Verification items for the finished model (mm, model axes). A direction names the side the tool comes from. Coordinates: 2 decimals unless noted, no trailing zeros. Write each loop counter-clockwise with the first axis right and the second up, starting at its lowest first coordinate (ties: lowest second). Pieces come first, ordered by that corner, then holes. Notation, with made-up numbers: M 50.5,21.5 L 97.5,21.5 A12 cw 97.5,30.5 Z; hole C 41.5,76 d4. An arc over 180 degrees is marked long. Answer in a Markdown table with one row per item.
from build123d import *

# Parameters (mm, degrees)
SKETCH1_W               = 0.625
SKETCH1_H               = 3.375
CUT_REVOLVE1_START      = -4.0000001
CUT_REVOLVE1_OUTLINE_R  = 0.625
CUT_REVOLVE1_DEPTH      = 4.6250001
SKETCH1_4_W             = 0.625
SKETCH1_4_H             = 3.375
SKETCH1_4_H_2           = 0.625
CUT_EXTRUDE1_DEPTH      = 20.584751879
CUT_EXTRUDE1_DEPTH_BACK = 20.584751879


# Read off the part's stored shape, not the designer's step: Cut-Revolve1
with BuildPart() as part:
    # Sketch1 → Revolve1 (revolve)
    with BuildSketch(Plane.XY):
        Polygon((18.75, 4), (16.875, 4), (16.875, 0.625), (16.875, 0), (18.75, 0), align=None)
        with Locations((16.5625, 2.3125)):
            Rectangle(SKETCH1_W, SKETCH1_H)
        Polygon((-18.75, 4), (-18.75, 0), (-16.875, 0), (-16.875, 0.625), (-0.625, 0.625), (0, 0.625), (16.25, 0.625), (16.25, 4), align=None)
    revolve(axis=Axis((0, 0, 0), (-1, 0, 0)))

    # Cut-Revolve1 outline → Cut-Revolve1 (cut)
    with BuildSketch(Plane(origin=(0, 0, 0), x_dir=(1, 0, 0), z_dir=(0, 1, 0)).offset(CUT_REVOLVE1_START)):
        Circle(CUT_REVOLVE1_OUTLINE_R)
    extrude(amount=CUT_REVOLVE1_DEPTH, mode=Mode.SUBTRACT)

    # Sketch1_4 → Cut-Revolve2 (revolve, cut)
    with BuildSketch(Plane.XY):
        with Locations((16.5625, 2.3125)):
            Rectangle(SKETCH1_4_W, SKETCH1_4_H)
        with Locations((16.5625, 0.3125)):
            Rectangle(SKETCH1_4_W, SKETCH1_4_H_2)
        with Locations((16.5625, -0.3125)):
            Rectangle(SKETCH1_4_W, SKETCH1_4_H_2)
    cut_revolve2 = revolve(axis=Axis((16.25, -0.625, 0), (0, -1, 0)), mode=Mode.SUBTRACT)

    # Mirror1: Cut-Revolve2 across plane
    add(cut_revolve2.mirror(Plane(origin=(0, 0, 0), x_dir=(0, 0, 1), z_dir=(1, 0, 0))), mode=Mode.SUBTRACT)

    # Sketch2 → Cut-Extrude1 (cut, two sides: drawn at the far end of the back side and taken through both)
    with BuildSketch(Plane(origin=(0, 0, 0), x_dir=(1, 0, 0), z_dir=(0, 1, 0)).offset(-CUT_EXTRUDE1_DEPTH_BACK)):
        with BuildLine():
            ThreePointArc((-18.318365102, -4), (-18.641778961, -2.011610591), (-18.75, 0))
            Line((-18.75, 0), (-18.75, -4))
            Line((-18.75, -4), (-18.318365102, -4))
        make_face()
        with BuildLine():
            Line((-18.318365102, 4), (-18.75, 4))
            Line((-18.75, 4), (-18.75, 0))
            ThreePointArc((-18.75, 0), (-18.641778961, 2.011610591), (-18.318365102, 4))
        make_face()
        with BuildLine():
            Line((18.318365102, -4), (18.75, -4))
            Line((18.75, -4), (18.75, 0))
            ThreePointArc((18.75, 0), (18.641778961, -2.011610591), (18.318365102, -4))
        make_face()
        with BuildLine():
            ThreePointArc((18.318365102, 4), (18.641778961, 2.011610591), (18.75, 0))
            Line((18.75, 0), (18.75, 4))
            Line((18.75, 4), (18.318365102, 4))
        make_face()
    extrude(amount=CUT_EXTRUDE1_DEPTH + CUT_EXTRUDE1_DEPTH_BACK, mode=Mode.SUBTRACT)

    # Sketch3 → Revolve2 (revolve)
    with BuildSketch(Plane.XY):
        Polygon((-5.5, 4), (-5.5, 5), (-6.5, 5), (-7.5, 4), align=None)
    revolve(axis=Axis((0, 0, 0), (-1, 0, 0)))


solid = part.part
1) Tool access check on faces 3 (the face through (16.875, 0, 0)), 4 (the face through (-0.624, -2.028, -0.027)), 5 (the face through (15.626, 2.028, 0.027)). Record the directions out of +Z, -Z, +X, -X, +Y, -Y that give a thin tool (end or side, any length) a straight path to the whole face; none if there is none.
Response values:
| item | result |
|---|---|
| face 3 | none |
| face 4 | -Y |
| face 5 | +Y |
2) Sectioned sample at A-A (x = 10). Record the cut outline in (y, z) (3 decimals), then the cut area to 3 significant figures.
Response values:
| item | result |
|---|---|
| outline | C 0,0 d8; hole C 0,0 d1.25 |
| area | 49.0 mm² |
3) Thickness scan on L1, parallel to X at y = 2, z = 0 (3 decimals); L2, parallel to Y at x = 9.5, z = 0 (3 decimals); L3, parallel to X at y = -1.05, z = 0 (3 decimals). Record the ranges inside material, lowest first. Write a range as [from, to].
Response values:
| item | result |
|---|---|
| L1 | x = [-18.75, -16.875], [-15.625, 15.625], [16.875, 18.75] |
| L2 | y = [-4, -0.625], [0.625, 4] |
| L3 | x = [-18.75, -0.625], [0.625, 18.75] |
4) Depth check by flat-ended pin: pin 1 (0.8 mm diameter, centred on x = -16.25, z = 0, fed in from +Y) (3 decimals); pin 2 (0.8 mm diameter, centred on x = 0, z = 0, fed in from +Y); pin 3 (0.6 mm diameter, centred on x = 0, z = 0, fed in from -Y) (3 decimals). Enter the tip coordinate at first touch or a pass-through.
Response values:
| item | result |
|---|---|
| pin 1 | stops at y = -0.625 |
| pin 2 | stops at y = 4 |
| pin 3 | stops at y = 0.625 |
5) Release check for a two-part mould opening along Z. For faces 1 (the face through (-15.626, 2.028, 0.027)), 2 (the face through (-13.204, -0.867, 3.905)) record: +Z half, -Z half, draft (parallel to the pull), parting line (faces both ways), or undercut.
Response values:
| item | result |
|---|---|
| face 1 | undercut |
| face 2 | parting line |
6) Sectioned sample at B-B (y = 1.5). Give the number of separate pieces and of enclosed holes in the cut face, then the cut area to 3 significant figures.
Response values:
| item | result |
|---|---|
| separate pieces | 1 |
| enclosed holes | 2 |
| area | 277 mm² |
